The drawing under review shows one solid part. Ordinate dimensions are in mm from its lowest x, y, z. Coordinates: 2 decimals unless noted, no trailing zeros. Write each loop counter-clockwise with the first axis right and the second up, starting at its lowest first coordinate (ties: lowest second). Pieces come first, ordered by that corner, then holes.
Q1. Take a section at A-A (x = 38.1). Give the boundary of the cut face in (y, z), and give its area (3 significant figures).
Q2. Take a section at C-C (x = 60.5). Give the boundary of the cut face in (y, z) (3 decimals).
Q3. Take a section at B-B (z = 76.2). Give the boundary of the cut face in (x, y).
Q4. For probe 1 along X at (y, z) = (4.5, 107); probe 2 along Y at (x, z) = (32, 110.5); probe 3 along X at (y, z) = (11.25, 71.5), list the stretches that pass through material, from the lowest coordinate up.
Q5. Take a section at D-D (z = 36.5). Give the boundary of the cut face in (x, y).
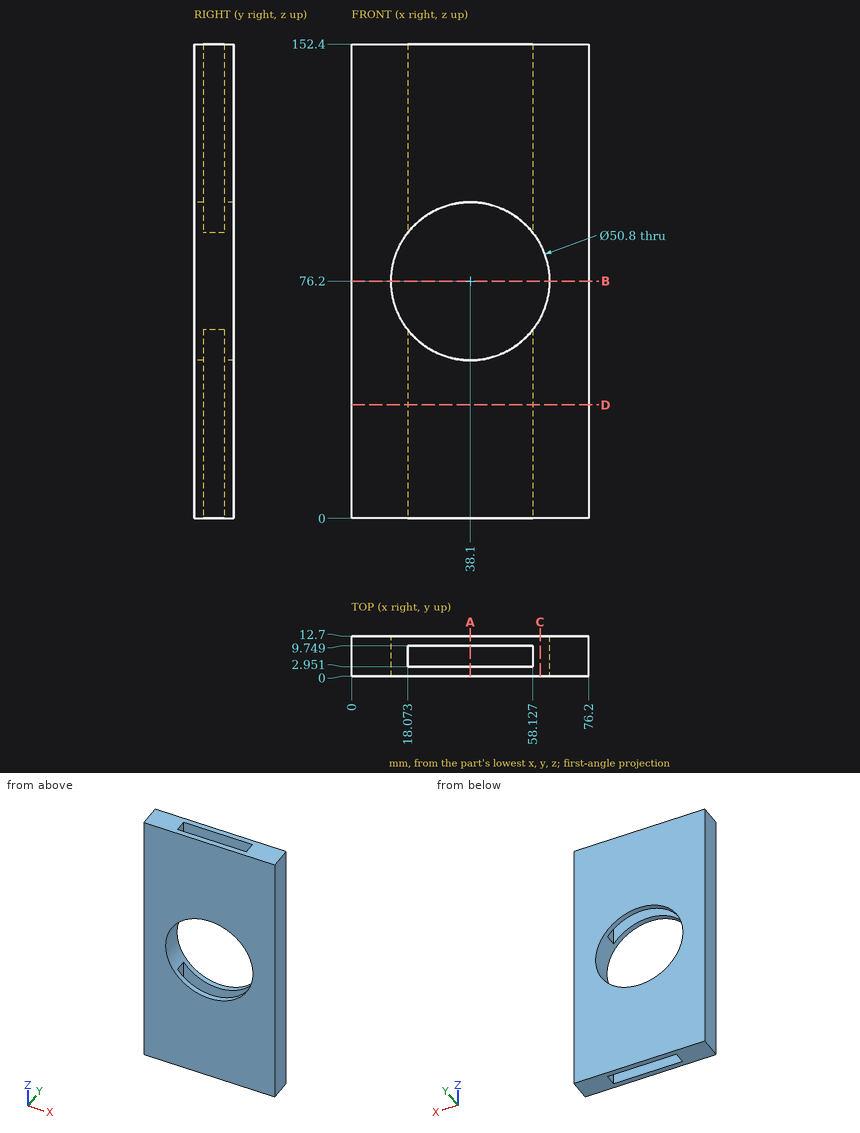
Response:
1. outline: (0, 0) - (2.95, 0) - (2.95, 50.8) - (0, 50.8) - close; (0, 101.6) - (2.95, 101.6) - (2.95, 152.4) - (0, 152.4) - close; (9.75, 0) - (12.7, 0) - (12.7, 50.8) - (9.75, 50.8) - close; (9.75, 101.6) - (12.7, 101.6) - (12.7, 152.4) - (9.75, 152.4) - close
1. area: 600 mm2
2. outline: (0, 0) - (12.7, 0) - (12.7, 64.225) - (0, 64.225) - close; (0, 88.175) - (12.7, 88.175) - (12.7, 152.4) - (0, 152.4) - close
3. outline: (0, 0) - (12.7, 0) - (12.7, 12.7) - (0, 12.7) - close; (63.5, 0) - (76.2, 0) - (76.2, 12.7) - (63.5, 12.7) - close
4. probe 1: x = 0 to 18.07, 58.13 to 76.2
4. probe 2: y = 0 to 2.95, 9.75 to 12.7
4. probe 3: x = 0 to 13.14, 63.06 to 76.2
5. outline: (0, 0) - (76.2, 0) - (76.2, 12.7) - (0, 12.7) - close; hole (18.07, 2.95) - (58.13, 2.95) - (58.13, 9.75) - (18.07, 9.75) - close
